Input: part model. Units: mm. Frame: model coordinates. A direction names the side the tool comes from. Coordinates: 2 decimals unless noted, no trailing zeros. Write each loop counter-clockwise with the first axis right and the second up, starting at its lowest first coordinate (ties: lowest second). Pieces come first, ordered by that corner, then holes. Notation, with made-up numbers: (88, 61.25) - (140, 61.25) arc R14 ccw to (140, 82.25) - close; hole circle Ø1 at (-22.75, 75). An arc over 180 degrees is marked (long way). Use a Markdown table: item, result. Add a question column.
Q1. Pin query (flat end, axial travel): P1, Ø0.9, axis at x = 32, z = 1, coming from the +Y side; P2, Ø0.9, axis at x = -16, z = 1.5, coming from the +Y side; P3, Ø0.9, axis at y = 1, z = 2, coming from the -X side. Return the tip coordinate at first contact, or that it passes through.
Q2. Section query A-A (x = -19.15). Return the cut outline in (y, z).
Q3. Set-up query: faces 1 (the face through (-16.81, 27.61, 1.48)), 2 (the face through (-34, 16.449, 1)), 3 (the face through (-17, 10.247, 2)), 4 (the face through (30, 0, 2)). Return all of +Z, -Z, +X, -X, +Y, -Y with unobstructed straight access to the full face (end or side cutting, diameter ignored); none if empty.
Q4. Section query C-C (y = 14.5). Return the cut outline in (x, z), then the cut area to 3 significant figures.
Q5. Section query B-B (z = 2.5). Give the number of separate pieces and of enclosed holes in the cut face, then the cut area to 3 significant figures.
Q6. Section query D-D (x = 9). Return the cut outline in (y, z).
Q7. Material intervals for probe 1 along X at (y, z) = (10.5, 0.95); probe 2 along Y at (x, z) = (25.4, 2.1); probe 3 along X at (y, z) = (-10, 0.75), sorted ascending. Write a range as from..to.
Q8. Mould query, pull axis Y, two halves, no side actions, for faces 5 (the face through (17, 10.247, 2)), 6 (the face through (-1, -3, 0)), 7 (the face through (16.98, 27.67, 1.48)), 8 (the face through (-19.42, -29.25, 1.52)). Classes: released by +Y, released by -Y, zero draft, split by the parting line, or undercut.
from build123d import *

# Parameters (mm, degrees)
BOSS_EXTRUDE1_DEPTH = 3
SKETCH2_R           = 1.5
CUT_EXTRUDE3_DEPTH  = 3
CUT_EXTRUDE4_START  = -10
CUT_EXTRUDE4_DEPTH  = 10
BOSS_EXTRUDE2_START = -3
BOSS_EXTRUDE2_DEPTH = 3
SKETCH5_W           = 0.56
SKETCH5_H           = 32.898596714
CUT_EXTRUDE5_DEPTH  = 3
SKETCH6_W           = 0.2
SKETCH6_H           = 32.898596714
CUT_EXTRUDE6_DEPTH  = 3
SKETCH7_R           = 2
CUT_EXTRUDE8_DEPTH  = 3
BOSS_EXTRUDE3_START = -3
BOSS_EXTRUDE3_DEPTH = 3
CUT_EXTRUDE9_START  = -3
CUT_EXTRUDE9_DEPTH  = 3
BOSS_EXTRUDE5_START = -3
BOSS_EXTRUDE5_DEPTH = 3
SKETCH11_R          = 1.5
CUT_EXTRUDE10_DEPTH = 3
CUT_EXTRUDE11_DEPTH = 3
SKETCH13_W          = 7
SKETCH13_H          = 1.5
CUT_EXTRUDE12_DEPTH = 3
SKETCH14_R          = 1.5
CUT_EXTRUDE13_DEPTH = 3


with BuildPart() as part:
    # Sketch1 → Boss-Extrude1 (new body)
    with BuildSketch(Plane.XY):
        with BuildLine():
            Line((-11, 25.5), (-22.790038711, 29.780264196))
            ThreePointArc((-22.790038711, 29.780264196), (0, -37.5), (22.790038711, 29.780264196))
            Line((22.790038711, 29.780264196), (11, 25.5))
            Line((11, 25.5), (-11, 25.5))
        make_face()
    extrude(amount=BOSS_EXTRUDE1_DEPTH)

    # Sketch2 → Cut-Extrude3 (cut)
    with BuildSketch(Plane.XY.offset(3)):
        with Locations((-25.400000001, 10.496905453)):
            Circle(SKETCH2_R)
        with Locations((-25.399981845, -10.493094547)):
            Circle(SKETCH2_R)
        with Locations(Location((25.399981845, -10.493094547, 0), (0, 0, 180))):
            Circle(SKETCH2_R)
        with Locations(Location((25.400000001, 10.496905453, 0), (0, 0, 180))):
            Circle(SKETCH2_R)
    extrude(amount=-CUT_EXTRUDE3_DEPTH, mode=Mode.SUBTRACT)

    # Sketch3 → Cut-Extrude4 (cut)
    with BuildSketch(Plane.XY.offset(3).offset(CUT_EXTRUDE4_START)):
        with BuildLine():
            Line((-30.76, 21.449298357), (-30.76, -21.449298357))
            ThreePointArc((-30.76, -21.449298357), (-37.5, 0), (-30.76, 21.449298357))
        make_face()
        with BuildLine():
            Line((30.76, 21.449298357), (30.76, -21.449298357))
            ThreePointArc((30.76, -21.449298357), (37.5, 0), (30.76, 21.449298357))
        make_face()
    extrude(amount=CUT_EXTRUDE4_DEPTH, mode=Mode.SUBTRACT)

    # Sketch4 → Boss-Extrude2 (add)
    with BuildSketch(Plane.XY.offset(3).offset(BOSS_EXTRUDE2_START)):
        with BuildLine():
            Line((-30.76, -21.449298357), (-30.76, -16.449298357))
            Line((-30.76, -16.449298357), (-33.699711921, -16.449298357))
            ThreePointArc((-33.699711921, -16.449298357), (-32.32667034, -19.006219634), (-30.76, -21.449298357))
        make_face()
        with BuildLine():
            Line((-33.699711921, 16.449298357), (-30.76, 16.449298357))
            Line((-30.76, 16.449298357), (-30.76, 21.449298357))
            ThreePointArc((-30.76, 21.449298357), (-32.32667034, 19.006219634), (-33.699711921, 16.449298357))
        make_face()
        with BuildLine():
            Line((30.76, 21.449298357), (30.76, 16.449298357))
            Line((30.76, 16.449298357), (33.699711921, 16.449298357))
            ThreePointArc((33.699711921, 16.449298357), (32.32667034, 19.006219634), (30.76, 21.449298357))
        make_face()
        with BuildLine():
            Line((30.76, -16.449298357), (30.76, -21.449298357))
            ThreePointArc((30.76, -21.449298357), (32.32667034, -19.006219634), (33.699711921, -16.449298357))
            Line((33.699711921, -16.449298357), (30.76, -16.449298357))
        make_face()
    extrude(amount=BOSS_EXTRUDE2_DEPTH)

    # Sketch5 → Cut-Extrude5 (cut)
    with BuildSketch(Plane.XY.offset(3)):
        with Locations((-30.48, 0)):
            Rectangle(SKETCH5_W, SKETCH5_H)
        with Locations((30.48, 0)):
            Rectangle(SKETCH5_W, SKETCH5_H)
    extrude(amount=-CUT_EXTRUDE5_DEPTH, mode=Mode.SUBTRACT)

    # Sketch6 → Cut-Extrude6 (cut)
    with BuildSketch(Plane.XY.offset(3)):
        with Locations((-30.1, 0)):
            Rectangle(SKETCH6_W, SKETCH6_H)
        with Locations((30.1, 0)):
            Rectangle(SKETCH6_W, SKETCH6_H)
    extrude(amount=-CUT_EXTRUDE6_DEPTH, mode=Mode.SUBTRACT)

    # Sketch7 → Cut-Extrude8 (cut)
    with BuildSketch(Plane.XY.offset(3)):
        with Locations((-19.15, -21.55)):
            Circle(SKETCH7_R)
        with Locations(Location((19.15, -21.55, 0), (0, 0, 180))):
            Circle(SKETCH7_R)
    extrude(amount=-CUT_EXTRUDE8_DEPTH, mode=Mode.SUBTRACT)

    # Sketch8 → Boss-Extrude3 (add)
    with BuildSketch(Plane.XY.offset(3).offset(BOSS_EXTRUDE3_START)):
        with BuildLine():
            Line((-33.699711921, 16.449298357), (-37.299711921, 16.449298357))
            ThreePointArc((-37.299711921, 16.449298357), (-32.744884003, 23.851322108), (-26.390038711, 29.780264196))
            Line((-26.390038711, 29.780264196), (-22.790038711, 29.780264196))
            ThreePointArc((-22.790038711, 29.780264196), (-29.020710607, 23.749702226), (-33.699711921, 16.449298357))
        make_face()
        with BuildLine():
            Line((33.699711921, 16.449298357), (37.299711921, 16.449298357))
            ThreePointArc((37.299711921, 16.449298357), (32.744884003, 23.851322108), (26.390038711, 29.780264196))
            Line((26.390038711, 29.780264196), (22.790038711, 29.780264196))
            ThreePointArc((22.790038711, 29.780264196), (29.020710607, 23.749702226), (33.699711921, 16.449298357))
        make_face()
    extrude(amount=BOSS_EXTRUDE3_DEPTH)

    # Sketch9 → Cut-Extrude9 (cut)
    with BuildSketch(Plane.XY.offset(3).offset(CUT_EXTRUDE9_START)):
        with BuildLine():
            Line((4.733920151, -37.2), (-4.733920151, -37.2))
            ThreePointArc((-4.733920151, -37.2), (0, -37.5), (4.733920151, -37.2))
        make_face()
    extrude(amount=CUT_EXTRUDE9_DEPTH, mode=Mode.SUBTRACT)

    # Sketch10 → Boss-Extrude5 (add)
    with BuildSketch(Plane.XY.offset(3).offset(BOSS_EXTRUDE5_START)):
        with BuildLine():
            ThreePointArc((-4.733920151, -37.2), (-21.838816892, -30.484685938), (-33.699711921, -16.449298357))
            Line((-33.699711921, -16.449298357), (-37.299711921, -16.449298357))
            ThreePointArc((-37.299711921, -16.449298357), (-23.43831182, -30.624902723), (-4.733920151, -37.2))
        make_face()
        with BuildLine():
            ThreePointArc((33.699711921, -16.449298357), (21.838816892, -30.484685938), (4.733920151, -37.2))
            ThreePointArc((4.733920151, -37.2), (23.43831182, -30.624902723), (37.299711921, -16.449298357))
            Line((37.299711921, -16.449298357), (33.699711921, -16.449298357))
        make_face()
        with BuildLine():
            Line((4.733920151, -37.2), (-4.733920151, -37.2))
            ThreePointArc((-4.733920151, -37.2), (0, -37.457659609), (4.733920151, -37.2))
        make_face()
    extrude(amount=BOSS_EXTRUDE5_DEPTH)

    # Sketch11 → Cut-Extrude10 (cut)
    with BuildSketch(Plane.XY.offset(3)):
        with Locations((-28.590038711, 23.780264196)):
            Circle(SKETCH11_R)
        with Locations(Location((28.590038711, 23.780264196, 0), (0, 0, 180))):
            Circle(SKETCH11_R)
    extrude(amount=-CUT_EXTRUDE10_DEPTH, mode=Mode.SUBTRACT)

    # Sketch12 → Cut-Extrude11 (cut)
    with BuildSketch(Plane.XY.offset(3)):
        Polygon((-22.005113558, -26.391105244), (-15.660959049, -29.349433076), (-16.294886442, -30.708894756), (-22.639040951, -27.750566924), align=None)
        Polygon((22.005113558, -26.391105244), (15.660959049, -29.349433076), (16.294886442, -30.708894756), (22.639040951, -27.750566924), align=None)
    extrude(amount=-CUT_EXTRUDE11_DEPTH, mode=Mode.SUBTRACT)

    # Sketch13 → Cut-Extrude12 (cut)
    with BuildSketch(Plane.XY.offset(3)):
        with Locations((-17.400000001, 9.496905453)):
            Rectangle(SKETCH13_W, SKETCH13_H)
        with Locations((17.400000001, 9.496905453)):
            Rectangle(SKETCH13_W, SKETCH13_H)
    extrude(amount=-CUT_EXTRUDE12_DEPTH, mode=Mode.SUBTRACT)

    # Sketch14 → Cut-Extrude13 (cut)
    with BuildSketch(Plane.XY.offset(3)):
        with Locations((-31.299711921, -19.449298357)):
            Circle(SKETCH14_R)
        with Locations((31.299711921, -19.449298357)):
            Circle(SKETCH14_R)
    extrude(amount=-CUT_EXTRUDE13_DEPTH, mode=Mode.SUBTRACT)


solid = part.part
Values follow:
| question | item | result |
|---|---|---|
| 1 | P1 | y = 25.23 |
| 1 | P2 | y = 27.48 |
| 1 | P3 | x = -30 |
| 2 | outline | (-33.03, 0) - (-29.38, 0) - (-29.38, 3) - (-33.03, 3) - close; (-27.72, 0) - (-23.55, 0) - (-23.55, 3) - (-27.72, 3) - close; (-19.55, 0) - (8.75, 0) - (8.75, 3) - (-19.55, 3) - close; (10.25, 0) - (28.46, 0) - (28.46, 3) - (10.25, 3) - close |
| 3 | face 1 | +Z, -Z, +Y |
| 3 | face 2 | +Z, -Z, -X |
| 3 | face 3 | +Z, -Z |
| 3 | face 4 | +Z, -Z, +X |
| 4 | outline | (-30, 0) - (30, 0) - (30, 3) - (-30, 3) - close |
| 4 | area | 180 mm2 |
| 5 | separate pieces | 1 |
| 5 | enclosed holes | 14 |
| 5 | area | 3,690 mm2 |
| 6 | outline | (-36.52, 0) - (25.5, 0) - (25.5, 3) - (-36.52, 3) - close |
| 7 | probe 1 | -30..-26.9, -23.9..23.9, 26.9..30 |
| 7 | probe 2 | -29.3..-11.99, -8.99..9, 12..29.78 |
| 7 | probe 3 | -30..-26.82, -23.98..23.98, 26.82..30 |
| 8 | face 5 | undercut |
| 8 | face 6 | zero draft |
| 8 | face 7 | released by +Y |
| 8 | face 8 | undercut |
